Source: CAD feature listing. Evaluate the final solid. Frame: model axes, mm. Give positions to 0.01 mm unless a question says otherwise; leave off trailing zeros. Order: outer loops, then holes, each group sorted by start corner. A loop starts at its lowest first (then second) coordinate and runs counter-clockwise, first axis right, second up. Notation, with made-up numbers: M -38,-10 L -14,-10 A7 ccw -14,-5 Z; hole C 18.5,14.25 d9. An arc over 180 degrees is marked long. Use CSV: the item, a comma, the result in double quotes. Start each with the question number.
1. Section query A-A, the plane x = 159. Return the cut outline in (y, z).
2. Pin query (flat end, axial travel): P1, Ø9.5, axis at x = 100, z = 7, coming from the -Y side; P2, Ø3, axis at y = 226.5, z = 13, coming from the +X side; P3, Ø5.5, axis at x = 204.5, y = 600, coming from the -Z side. Return the tip coordinate at first contact, or that it passes through.
3. Line query: line 1 along Y through (x, z) = (313, 6); line 2 along Y through (x, z) = (144.5, 10.75); line 3 along X through (y, z) = (239.5, 12.75). Output: solid intervals per line, ascending. Write a range as [from, to].
Autodesk Fusion 360 part; units mm, degrees
sketch "Sketch2" plane through (0, 0, 0) normal (0, 0, 1) x (1, 0, 0)
  line L0 (0, 0) -> (376.7667, 0)
  line L1 (376.7667, 0) -> (376.7667, 609.6)
  line L2 (376.7667, 609.6) -> (0, 609.6)
  line L3 (0, 609.6) -> (0, 0)
  dimension "d4" = 376.7667
  dimension "d5" = 609.6
extrude "Extrude1" add sketch "Sketch2" along normal blind 19.05
sketch "Sketch3" plane through (0, 0, 19.05) normal (0, 0, 1) x (-1, 0, 0)
  line L0 (0, -609.6) -> (0, 0)
  line L1 (0, 0) -> (-376.7667, 0)
  line L2 (-376.7667, 0) -> (-376.7667, -609.6)
  line L3 (-376.7667, -609.6) -> (0, -609.6)
  line L4 (25.4, 0) -> (402.1667, 0)
  line L5 (402.1667, 0) -> (402.1667, -376.7667)
  line L6 (402.1667, -376.7667) -> (25.4, -376.7667)
  line L7 (25.4, -376.7667) -> (25.4, 0)
  dimension "d8" = 376.7667
  dimension "d9" = 376.7667
sketch "Sketch4" plane through (0, 0, 19.05) normal (0, 0, 1) x (-1, 0, 0)
  line L0 (0, -609.6) -> (0, 0)
  line L1 (0, 0) -> (-376.7667, 0)
  line L2 (-376.7667, 0) -> (-376.7667, -609.6)
  line L3 (-376.7667, -609.6) -> (0, -609.6)
  line L4 (25.4, 0) -> (71.9667, 0)
  line L5 (25.4, 0) -> (25.4, -25.4)
  line L6 (402.1667, -25.4) -> (402.1667, 0)
  line L7 (402.1667, -25.4) -> (402.1667, 0)
  line L8 (46.587, 0) -> (25.4, 0)
  line L9 (71.9667, 0) -> (56.4444, 0)
  line L10 (56.4444, 0) -> (71.9667, -25.4)
  line L11 (150.9889, 0) -> (135.4667, -25.4)
  line L12 (150.9889, 0) -> (166.5111, 0)
  line L13 (166.5111, 0) -> (182.0333, 0)
  line L14 (166.5111, 0) -> (182.0333, -25.4)
  line L15 (245.5333, -25.4) -> (261.0555, 0)
  line L16 (261.0555, 0) -> (276.5778, 0)
  line L17 (276.5778, 0) -> (292.1, -25.4)
  line L18 (355.6, -25.4) -> (371.1222, 0)
  line L19 (402.1667, 0) -> (386.6444, 0)
  line L20 (386.6444, 0) -> (371.1222, 0)
  line L21 (402.1667, 0) -> (402.1667, -376.7667)
  line L22 (402.1667, -188.3833) -> (25.4, -188.3833)
  line L23 (402.1667, -351.3667) -> (402.1667, -376.7667)
  line L24 (402.1667, -376.7667) -> (402.1667, 0)
  line L25 (166.5111, -376.7667) -> (182.0333, -376.7667)
  line L26 (386.6444, -376.7667) -> (371.1222, -376.7667)
  line L27 (25.4, -376.7667) -> (71.9667, -376.7667)
  line L28 (166.5111, -376.7667) -> (182.0333, -351.3667)
  line L29 (355.6, -351.3667) -> (371.1222, -376.7667)
  line L30 (402.1667, -351.3667) -> (402.1667, -376.7667)
  line L31 (56.4444, -376.7667) -> (71.9667, -351.3667)
  line L32 (245.5333, -351.3667) -> (261.0555, -376.7667)
  line L33 (25.4, -376.7667) -> (25.4, -351.3667)
  line L34 (261.0555, -376.7667) -> (276.5778, -376.7667)
  line L35 (71.9667, -376.7667) -> (56.4444, -376.7667)
  line L36 (46.587, -376.7667) -> (25.4, -376.7667)
  line L37 (276.5778, -376.7667) -> (292.1, -351.3667)
  line L38 (402.1667, -376.7667) -> (386.6444, -376.7667)
  line L39 (150.9889, -376.7667) -> (166.5111, -376.7667)
  line L40 (150.9889, -376.7667) -> (135.4667, -351.3667)
  line L41 (25.4, -25.4) -> (25.4, -19.05)
  line L42 (25.4, -19.05) -> (414.4129, -19.05)
  line L43 (402.1667, -351.3667) -> (402.1667, -357.7167)
  line L44 (402.1667, -357.7167) -> (12.7, -357.7167)
  dimension "d12" = 46.5667
  dimension "d13" = 25.4
  dimension "d14" = 376.7667
  dimension "d15" = 46.5667
  dimension "d16" = 63.5
  dimension "d17" = 46.5667
  dimension "d18" = 15.5222
  dimension "d20" = 15.5222
  dimension "d21" = 15.5222
  dimension "d22" = 63.5
  dimension "d24" = 46.5667
  dimension "d25" = 15.5222
  dimension "d26" = 63.5
  dimension "d456" = 376.7667
  dimension "d473" = 6.35
  dimension "d474" = 6.35
sketch "Sketch5" plane through (0, 609.6, 0) normal (0, 1, 0) x (-1, 0, 0)
  line L0 (-376.7667, 0) -> (0, 0)
  line L1 (0, 0) -> (0, 19.05)
  line L2 (0, 19.05) -> (-376.7667, 19.05)
  line L3 (-376.7667, 19.05) -> (-376.7667, 0)
  line L4 (-376.7667, 0) -> (0, 0)
  line L5 (-123.6562, -70.3757) -> (-108.134, -95.7757)
  line L6 (-328.2673, -70.3757) -> (-343.7895, -70.3757)
  line L7 (-343.7895, -70.3757) -> (-328.2673, -95.7757)
  line L8 (-154.7007, -95.7757) -> (-139.1784, -70.3757)
  line L9 (-233.7229, -70.3757) -> (-218.2007, -95.7757)
  line L10 (-374.834, -95.7757) -> (-328.2673, -95.7757)
  line L11 (-139.1784, -70.3757) -> (-123.6562, -70.3757)
  line L12 (-233.7229, -70.3757) -> (-218.2007, -70.3757)
  line L13 (-249.2451, -70.3757) -> (-264.7673, -95.7757)
  line L14 (-13.5895, -70.3757) -> (-29.1118, -70.3757)
  line L15 (-44.634, -95.7757) -> (-29.1118, -70.3757)
  line L16 (1.9327, -70.3757) -> (-13.5895, -70.3757)
  line L17 (1.9327, -95.7757) -> (1.9327, -70.3757)
  line L18 (-328.2673, -70.3757) -> (-249.2451, -70.3757)
  line L19 (-264.7673, -95.7757) -> (-328.2673, -95.7757)
  line L20 (-218.2007, -95.7757) -> (-154.7007, -95.7757)
  line L21 (-108.134, -95.7757) -> (-44.634, -95.7757)
  line L22 (-29.1118, -70.3757) -> (-123.6562, -70.3757)
  line L23 (-139.1784, -70.3757) -> (-233.7229, -70.3757)
  dimension "d463" = 63.5
  dimension "d464" = 46.5667
  dimension "d465" = 15.5222
  dimension "d466" = 15.5222
  dimension "d467" = 15.5222
  dimension "d468" = 63.5
  dimension "d469" = 46.5667
  dimension "d470" = 15.5222
  dimension "d471" = 63.5
sketch "Sketch6" plane through (0, 0, 0) normal (0, -1, 0) x (1, 0, 0)
  line L0 (0, 0) -> (376.7667, 0)
  line L1 (376.7667, 0) -> (376.7667, 19.05)
  line L2 (376.7667, 19.05) -> (0, 19.05)
  line L3 (0, 19.05) -> (0, 0)
  line L4 (46.5667, 19.05) -> (31.0444, 19.05)
  line L5 (0, -6.35) -> (0, 0)
  line L6 (361.2444, 19.05) -> (345.7222, 19.05)
  line L7 (376.7667, -6.35) -> (376.7667, 19.05)
  line L8 (31.0444, 19.05) -> (46.5667, -6.35)
  line L9 (235.6555, 19.05) -> (251.1778, 19.05)
  line L10 (125.5889, 19.05) -> (141.1111, 19.05)
  line L11 (330.2, -6.35) -> (345.7222, 19.05)
  line L12 (0, 0) -> (389.0129, 0)
  line L13 (125.5889, 19.05) -> (110.0667, -6.35)
  line L14 (376.7667, -6.35) -> (376.7667, 19.05)
  line L15 (376.7667, 19.05) -> (361.2444, 19.05)
  line L16 (0, 19.05) -> (0, -6.35)
  line L17 (0, 19.05) -> (46.5667, 19.05)
  line L18 (220.1333, -6.35) -> (235.6555, 19.05)
  line L19 (21.187, 19.05) -> (0, 19.05)
  line L20 (141.1111, 19.05) -> (156.6333, -6.35)
  line L21 (141.1111, 19.05) -> (156.6333, 19.05)
  line L22 (251.1778, 19.05) -> (266.7, -6.35)
  point P0 (376.7667, 19.05)
  dimension "d492" = 46.5667
  dimension "d493" = 25.4
  dimension "d494" = 376.7667
  dimension "d495" = 46.5667
  dimension "d496" = 63.5
  dimension "d497" = 46.5667
  dimension "d498" = 15.5222
  dimension "d499" = 15.5222
  dimension "d500" = 15.5222
  dimension "d501" = 63.5
  dimension "d502" = 46.5667
  dimension "d503" = 15.5222
  dimension "d504" = 63.5
  dimension "d505" = 6.35
fillet "Fillet2" radius 6.35 4 edges at (376.7667, 0, 9.525) (0, 0, 9.525) (376.7667, 609.6, 9.525) (0, 609.6, 9.525)
fillet "Fillet3" radius 8.382 8 edges at (374.9068, 607.7401, 19.05) (188.3833, 609.6, 19.05) (1.8599, 607.7401, 19.05) (0, 304.8, 19.05) (1.8599, 1.8599, 19.05) (188.3833, 0, 19.05) (374.9068, 1.8599, 19.05) (376.7667, 304.8, 19.05)
extrude "Extrude6" cut sketch "Sketch6" against normal blind 19.05 contours L0 L2 L4 L8 L12 L13 L17 | L0 L2 L12 L18 L20 L21 | L0 L2 L11 L12 L22
sketch "Sketch7" plane through (0, 609.6, 0) normal (0, 1, 0) x (-1, 0, 0)
  line L0 (-370.4167, 0) -> (-6.35, 0)
  line L1 (0, 19.05) -> (-376.7667, 19.05)
  line L2 (-376.7667, 19.05) -> (-376.7667, 0)
  line L3 (-355.5797, 19.05) -> (-376.7667, 19.05)
  line L4 (-376.7667, 19.05) -> (-376.7667, -6.35)
  line L5 (-345.7222, 19.05) -> (-330.2, -6.35)
  line L6 (-376.7667, 19.05) -> (-330.2, 19.05)
  line L7 (-376.7667, 0) -> (0, 0)
  line L8 (-330.2, 19.05) -> (-345.7222, 19.05)
  line L9 (-156.6334, -6.35) -> (-141.1111, 19.05)
  line L10 (-251.1778, 19.05) -> (-266.7, -6.35)
  line L11 (-46.5667, -6.35) -> (-31.0445, 19.05)
  line L12 (-141.1111, 19.05) -> (-125.5889, 19.05)
  line L13 (-125.5889, 19.05) -> (-110.0667, -6.35)
  line L14 (-235.6556, 19.05) -> (-220.1333, 19.05)
  line L15 (-251.1778, 19.05) -> (-235.6556, 19.05)
  line L16 (-15.5222, 19.05) -> (-31.0445, 19.05)
  line L17 (0, -6.35) -> (0, 19.05)
  line L18 (0, -6.35) -> (0, 19.05)
  line L19 (-235.6556, 19.05) -> (-220.1334, -6.35)
  line L20 (0, 0) -> (0, 19.05)
  line L21 (0, 19.05) -> (-15.5222, 19.05)
  line L22 (0, 19.05) -> (0, 9.525)
  line L23 (-15.5222, 0) -> (-31.0445, 0)
  line L24 (-330.2, 0) -> (-345.7222, 0)
  line L25 (-235.6556, 0) -> (-220.1333, 0)
  line L26 (-376.7667, 0) -> (-330.2, 0)
  line L27 (-376.7667, 0) -> (-376.7667, 19.05)
  line L28 (-355.5797, 0) -> (-376.7667, 0)
  line L29 (-141.1111, 0) -> (-125.5889, 0)
  line L30 (0, 0) -> (-15.5222, 0)
  line L31 (-251.1778, 0) -> (-235.6556, 0)
  line L32 (0, 0) -> (0, 9.525)
  line L33 (-376.7667, 19.05) -> (0, 19.05)
  line L34 (0, 19.05) -> (0, 0)
  line L35 (-376.7667, 19.05) -> (0, 19.05)
  line L36 (-376.7667, 0) -> (-376.7667, 25.4)
  line L37 (0, 0) -> (-376.7667, 0)
  line L38 (-376.7667, 0) -> (-376.7667, 19.05)
  line L39 (0, 19.05) -> (0, 0)
  line L40 (0, 0) -> (-376.7667, 0)
  line L41 (-6.35, 10.668) -> (-370.4167, 10.668)
  line L42 (-370.4167, 10.668) -> (-370.4167, 0)
  line L43 (-6.35, 0) -> (-6.35, 10.668)
  point P0 (0, 19.05)
  point P1 (-376.7667, 0)
  point P2 (0, 0)
  point P3 (-376.7667, 19.05)
  point P4 (0, 19.05)
  dimension "d522" = 46.5667
  dimension "d523" = 25.4
  dimension "d524" = 376.7667
  dimension "d525" = 46.5667
  dimension "d526" = 63.5
  dimension "d527" = 46.5667
  dimension "d528" = 15.5222
  dimension "d529" = 15.5222
  dimension "d530" = 15.5222
  dimension "d531" = 63.5
  dimension "d532" = 46.5667
  dimension "d533" = 15.5222
  dimension "d534" = 63.5
extrude "Extrude7" cut sketch "Sketch7" against normal blind 19.05 contours L0 L5 L7 L10 L24 L26 L37 L40 L41 | L0 L7 L9 L19 L25 L37 L40 L41 | L0 L7 L11 L13 L37 L40 L41
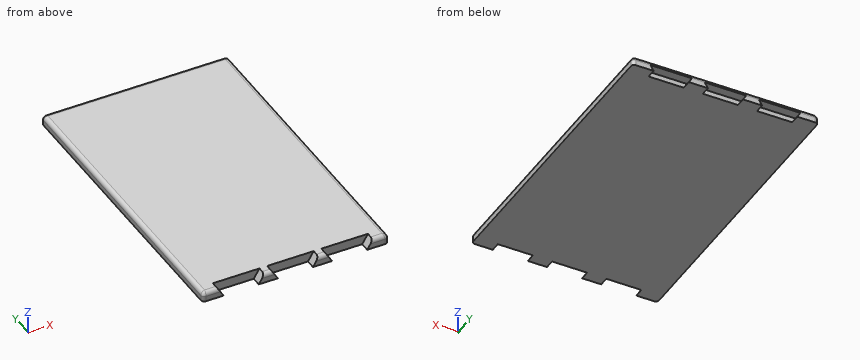
Result set:
1,outline,"M 19.05,0 L 590.55,0 L 590.55,10.67 L 609.6,10.67 A8.38 ccw 601.22,19.05 L 19.05,19.05 Z"
2,P1,"y = 19.05"
2,P2,"x = 376.73"
2,P3,"z = 10.67"
3,line 1,"[19.05, 590.55]"
3,line 2,"[0, 609.6]"
3,line 3,"[0.26, 376.5]"
